The listing builds one solid part. Answer for the finished solid, in the listing's coordinates (mm). A direction names the side the tool comes from. Round coordinates to 2 decimals unless told otherwise and drop trailing zeros. Write each loop counter-clockwise with the first axis right and the second up, starting at its lowest first coordinate (ties: lowest second). Pieces come first, ordered by that corner, then holes.
Item 1: Find section A-A on z = 1.6. Give the vertices of the cut face in (x, y), then the cut area to 3 significant figures.
Item 2: Each of these flat-tipped pins is pushed along its axis until it touches: pin 1 (5 mm diameter, centred on x = 18, y = 0, fed in from -Z); pin 2 (1 mm diameter, centred on y = 3, z = 1, fed in from -X); pin 3 (0.6 mm diameter, centred on x = 1.5, z = 1.5, fed in from +Y); pin 4 (0.6 mm diameter, centred on y = 5, z = 0.5, fed in from +X). Where does it stop, or does it pass through?
Item 3: Find section C-C on y = 0. Give the vertices of the cut face in (x, z), then the cut area to 3 significant figures.
Item 4: Find section B-B on x = 0. Give the vertices of the cut face in (y, z), then the cut area to 3 significant figures.
Item 5: A tool of negligible diameter and unlimited length cuts with its end or side. For faces 4 (the face through (5.2, 0.4, 0)), 5 (the face through (0, 10, 1)), from which of +Z, -Z, +X, -X, +Y, -Y can it reach the whole face along a straight path? Write none if from no direction.
Item 6: Find section D-D on y = -5. Give the vertices of the cut face in (x, z), then the cut area to 3 significant figures.
Item 7: For a pull along Y with two mould halves and no side action, classify faces 1 (the face through (0, -10, 1)), 2 (the face through (5.2, 0.4, 2)), 3 (the face through (23.846, 7.509, 0.986)) as +Y half, -Y half, draft (parallel to the pull), parting line (faces both ways), or undercut.
Item 8: Find the intervals of material crossed by probe 1 along Y at (x, z) = (3, 1.8); probe 2 along Y at (x, z) = (-17, 0.55); probe 3 along X at (y, z) = (-6, 0.6), in increasing order.
```python
from build123d import *

# Parameters (mm, degrees)
SKETCH1_R           = 25
BOSS_EXTRUDE1_DEPTH = 2
SKETCH2_W           = 10
SKETCH2_H           = 20
CUT_EXTRUDE1_DEPTH  = 5
SKETCH3_R           = 3
CUT_EXTRUDE2_DEPTH  = 5


with BuildPart() as part:
    # Sketch1 → Boss-Extrude1 (new body)
    with BuildSketch(Plane.XY):
        Circle(SKETCH1_R)
    extrude(amount=BOSS_EXTRUDE1_DEPTH)

    # Sketch2 → Cut-Extrude1 (cut)
    with BuildSketch(Plane.XY):
        Rectangle(SKETCH2_W, SKETCH2_H)
    extrude(amount=CUT_EXTRUDE1_DEPTH, mode=Mode.SUBTRACT)

    # Sketch3 → Cut-Extrude2 (cut)
    with BuildSketch(Plane.XY):
        with Locations((-18, 0)):
            Circle(SKETCH3_R)
        with Locations((18, 0)):
            Circle(SKETCH3_R)
    extrude(amount=CUT_EXTRUDE2_DEPTH, mode=Mode.SUBTRACT)


solid = part.part
```
Check values:
1. outline: circle Ø50 at (0, 0); hole circle Ø6 at (-18, 0); hole (-5, -10) - (5, -10) - (5, 10) - (-5, 10) - close; hole circle Ø6 at (18, 0)
1. area: 1,710 mm2
2. pin 1: passes through
2. pin 2: stops at x = -24.87
2. pin 3: stops at y = 24.97
2. pin 4: stops at x = 24.55
3. outline: (-25, 0) - (-21, 0) - (-21, 2) - (-25, 2) - close; (-15, 0) - (-5, 0) - (-5, 2) - (-15, 2) - close; (5, 0) - (15, 0) - (15, 2) - (5, 2) - close; (21, 0) - (25, 0) - (25, 2) - (21, 2) - close
3. area: 56.0 mm2
4. outline: (-25, 0) - (-10, 0) - (-10, 2) - (-25, 2) - close; (10, 0) - (25, 0) - (25, 2) - (10, 2) - close
4. area: 60.0 mm2
5. face 4: -Z, +X, -X, +Y, -Y
5. face 5: +Z, -Z
6. outline: (-24.49, 0) - (-5, 0) - (-5, 2) - (-24.49, 2) - close; (5, 0) - (24.49, 0) - (24.49, 2) - (5, 2) - close
6. area: 78.0 mm2
7. face 1: undercut
7. face 2: draft
7. face 3: parting line
8. probe 1: y = -24.82 to -10, 10 to 24.82
8. probe 2: y = -18.33 to -2.83, 2.83 to 18.33
8. probe 3: x = -24.27 to -5, 5 to 24.27
